```python
from build123d import *

# Parameters (mm, degrees)
F1_DEPTH = 2
F2_R     = 5
F3_R     = 1


with BuildPart() as f1:
    # F0 (on Top) → F1 (new body)
    with BuildSketch(Plane.XY):
        with BuildLine():
            Line((8.5, 8), (-8.5, 8))
            Line((-8.5, 8), (-8.5, 4.5))
            Line((-8.5, 4.5), (0, 4.5))
            ThreePointArc((0, 4.5), (3.181981, 3.181981), (4.5, 0))
            ThreePointArc((4.5, 0), (3.181981, -3.181981), (0, -4.5))
            Line((0, -4.5), (-8.5, -4.5))
            Line((-8.5, -4.5), (-8.5, -8))
            Line((-8.5, -8), (8.5, -8))
            Line((8.5, -8), (8.5, 8))
        make_face()
        with BuildLine():
            Line((0, 4.5), (-8.5, 4.5))
            Line((-8.5, 4.5), (-8.5, 4))
            Line((-8.5, 4), (-2.061553, 4))
            ThreePointArc((-2.061553, 4), (-1.06066, 4.373214), (0, 4.5))
        make_face()
        with BuildLine():
            Line((-2.061553, -4), (-8.5, -4))
            Line((-8.5, -4), (-8.5, -4.5))
            Line((-8.5, -4.5), (0, -4.5))
            ThreePointArc((0, -4.5), (-1.06066, -4.373214), (-2.061553, -4))
        make_face()
    extrude(amount=F1_DEPTH)

    # F2
    f2_edges = [f1.edges().sort_by_distance(p)[0] for p in [
        (8.5, 8, 1),
        (8.5, -8, 1),
    ]]
    fillet(f2_edges, radius=F2_R)

    # F3
    f3_edges = [f1.edges().sort_by_distance(p)[0] for p in [
        (-2.061553, -4, 1),
        (-2.061553, 4, 1),
        (-2.5, 8, 2),
        (-8.5, -4, 1),
        (-8.5, -8, 1),
        (-8.5, 4, 1),
        (-8.5, 8, 1),
    ]]
    fillet(f3_edges, radius=F3_R)


solid = f1.part
```
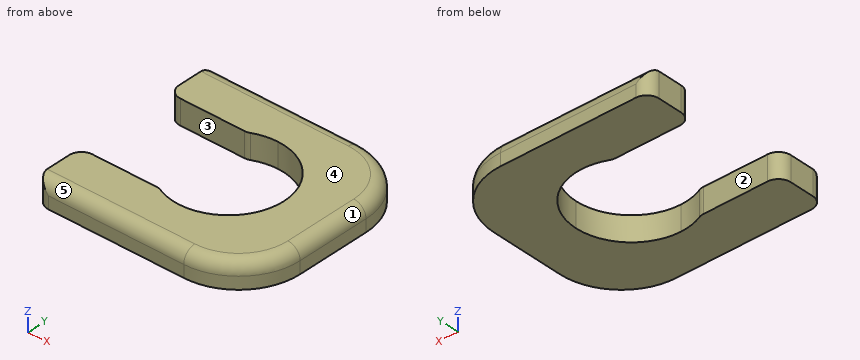
Build history of the part. All positions in model axes, mm. Face numbers are marked on the shaded views. A direction names the side the tool comes from. Give positions to 0.01 mm unless a question says otherwise; leave off trailing zeros. Loops run counter-clockwise (first coordinate to the right, second up) from the corner with the lowest first, then second, coordinate; pieces in that order, holes last. Notation, with made-up numbers: (48, -13.75) -> (95, -13.75) arc R29 cw to (95, 24.25) -> close; hole circle Ø8 at (55, -38.75). An arc over 180 degrees is marked (long way). One line per question, with ' | ' between items. Start each with the question number.
1) Pin check, flat tips, straight feed: pin 1 (6 mm diameter, centred on x = 3.5, y = 2.5, fed in from -Z); pin 2 (1 mm diameter, centred on y = -4.5, z = 1, fed in from +X). Stop position of each tip, or through.
2) Two-plate mould, pull along Y, no slides. Class the marked faces 3, 4 and 5: released by +Y, released by -Y, zero draft, split by the parting line, or undercut.
3) Probe L1, parallel to Y at x = -3.5, z = 0.25; L2, parallel to Y at x = 1.5, z = 1.35; L3, parallel to X at y = -6, z = 0.6. List the from-to ranges inside material, lowest first.
4) Cut at B-B (z = 1.8). Give the cut face in (x, y), plus the area to 3 significant figures.
5) Cut at D-D (z = 0.2). Give the cut face in (x, y), plus the area to 3 significant figures.
6) Cut at C-C (y = 1.5). Give the cut face in (x, z), plus the area to 3 significant figures.
7) 3-axis set-ups, long thin cutter, end or side, ignore diameter. For the marked faces 1 and 2: which of +Z, -Z, +X, -X, +Y, -Y reach the whole face in a straight line?
8) Cut at A-A (x = 3.25). Give the cut face in (y, z).
Return value:
1) pin 1: z = 0 | pin 2: x = 8.4
2) face 3: undercut | face 4: zero draft | face 5: released by -Y
3) L1: -8 to -4, 4 to 8 | L2: -7.94 to -4.24, 4.24 to 7.94 | L3: -8.5 to 7.5
4) outline: (-8.5, -7) arc R1 ccw to (-8.3, -7.6) -> (3.5, -7.6) arc R4.6 ccw to (8.1, -3) -> (8.1, 3) arc R4.6 ccw to (3.5, 7.6) -> (-8.3, 7.6) arc R1 ccw to (-8.5, 7) -> (-8.5, 5) arc R1 ccw to (-7.5, 4) -> (-2.29, 4) arc R1 ccw to (-1.87, 4.09) arc R4.5 cw to (0, 4.5) arc R4.5 cw to (4.5, 0) arc R4.5 cw to (0, -4.5) arc R4.5 cw to (-1.87, -4.09) arc R1 ccw to (-2.29, -4) -> (-7.5, -4) arc R1 ccw to (-8.5, -5) -> close | area: 142 mm^2
5) outline: (-8.5, -7) arc R1 ccw to (-7.5, -8) -> (3.5, -8) arc R5 ccw to (8.5, -3) -> (8.5, 3) arc R5 ccw to (3.5, 8) -> (-7.5, 8) arc R1 ccw to (-8.5, 7) -> (-8.5, 5) arc R1 ccw to (-7.5, 4) -> (-2.29, 4) arc R1 ccw to (-1.87, 4.09) arc R4.5 cw to (0, 4.5) arc R4.5 cw to (4.5, 0) arc R4.5 cw to (0, -4.5) arc R4.5 cw to (-1.87, -4.09) arc R1 ccw to (-2.29, -4) -> (-7.5, -4) arc R1 ccw to (-8.5, -5) -> close | area: 159 mm^2
6) outline: (4.24, 0) -> (8.5, 0) -> (8.5, 1) arc R1 ccw to (7.5, 2) -> (4.24, 2) -> close | area: 8.30 mm^2
7) face 1: +Z, +X, +Y, -Y | face 2: +Z, -Z, -X
8) outline: (-8, 0) -> (-3.11, 0) -> (-3.11, 2) -> (-7, 2) arc R1 ccw to (-8, 1) -> close; (3.11, 0) -> (8, 0) -> (8, 1) arc R1 ccw to (7, 2) -> (3.11, 2) -> close
